Autodesk Inventor part; units mm, degrees
ref_plane "YZ Plane" through (0, 0, 0) normal (1, 0, 0) x (0, 1, 0)
ref_plane "XZ Plane" through (0, 0, 0) normal (0, 1, 0) x (-1, 0, 0)
ref_plane "XY Plane" through (0, 0, 0) normal (0, 0, 1) x (1, 0, 0)
sketch "Sketch1" plane through (0, 0, 0) normal (1, 0, 0) x (0, 1, 0)
  line L0 (13.5, 0) -> (169.5, 0)
  line L1 (183, -13.5) -> (183, -169.5)
  line L2 (169.5, -183) -> (13.5, -183)
  line L3 (0, -169.5) -> (0, -13.5)
  arc A0 (183, -13.5) -> (169.5, 0) centre (169.5, -13.5) ccw
  arc A1 (169.5, -183) -> (183, -169.5) centre (169.5, -169.5) ccw
  arc A2 (0, -169.5) -> (13.5, -183) centre (13.5, -169.5) ccw
  arc A3 (13.5, 0) -> (0, -13.5) centre (13.5, -13.5) ccw
  line L4 (169.5, -13.5) -> (13.5, -13.5)
  line L5 (13.5, -13.5) -> (13.5, -145.5)
  line L6 (37.5, -169.5) -> (169.5, -169.5)
  line L7 (169.5, -169.5) -> (169.5, -13.5)
  line L8 (169.5, -13.5) -> (179.0459, -3.9541) construction
  line L9 (169.5, -169.5) -> (179.0459, -179.0459) construction
  line L10 (13.5, -13.5) -> (3.9541, -3.9541) construction
  line L11 (33.0959, -149.5) -> (0, -149.5) construction
  line L12 (33.5, -149.9041) -> (33.5, -183) construction
  circle A4 centre (6.0754, -6.0754) radius 3 construction
  circle A5 centre (6.0754, -6.0754) radius 1.1
  circle A6 centre (176.9246, -6.0754) radius 3 construction
  circle A7 centre (176.9246, -6.0754) radius 1.1
  circle A8 centre (176.9246, -176.9246) radius 3 construction
  circle A9 centre (176.9246, -176.9246) radius 1.1
  circle A10 centre (33.5, -180) radius 3 construction
  circle A11 centre (33.5, -180) radius 1.1
  circle A12 centre (3, -149.5) radius 3 construction
  circle A13 centre (3, -149.5) radius 1.1
  line L13 (13.5, -169.5) -> (24.5, -158.5) construction
  circle A14 centre (24.5, -158.5) radius 8.1
  line L14 (13.5, -145.5) -> (33.5, -145.5)
  line L15 (37.5, -149.5) -> (37.5, -169.5)
  arc A15 (37.5, -149.5) -> (33.5, -145.5) centre (33.5, -149.5) ccw
  point P0 (0, 0)
  point P1 (37.5, -145.5)
  dimension "d6" = 6
  dimension "d0" = 13.5
  dimension "d1" = 183
  dimension "d2" = 183
  dimension "d3" = 20
  dimension "d4" = 20
  dimension "d5" = 2.2
  dimension "d10" = 16.2
  dimension "d11" = 24.5
  dimension "d12" = 45
  dimension "d13" = 24
  dimension "d14" = 4
extrude "Extrusion1" add sketch "Sketch1" along normal blind 2.5
properties part number "FrontPanelSquishything"
Verification items for the finished model (mm, model axes). A direction names the side the tool comes from. Round coordinates to 2 decimals unless told otherwise and drop trailing zeros. Order: outer loops, then holes, each group sorted by start corner. A loop starts at its lowest first (then second) coordinate and runs counter-clockwise, first axis right, second up.
1) Draft check along Y on faces 1 (the flat face through (0, 90, -172)), 2 (the cylindrical face through (1.2, 28.9, -165.3)), 3 (the cylindrical face through (1.23, 4.06, -179.15)). Enter one of: +Y half, -Y half, draft (parallel to the pull), parting line (faces both ways), or undercut.
Geometry says:
face 1: draft
face 2: undercut
face 3: -Y half
2) Depth check by flat-ended pin: pin 1 (13 mm diameter, centred on y = 24.5, z = -158.5, fed in from +X). Enter the tip coordinate at first touch or a pass-through.
Geometry says:
pin 1: passes through
3) Material ranges on line 1 (Y direction, x = 0.3, z = -16.5); line 2 (Z direction, x = 2.3, y = 126); line 3 (Z direction, x = 1.25, y = 33.5), recorded low to high.
Geometry says:
line 1: y = 0 to 13.5, 169.5 to 183
line 2: z = -183 to -169.5, -13.5 to 0
line 3: z = -183 to -181.1, -178.9 to -145.5, -13.5 to 0
4) Cross-section at D-D, the plane y = 30. Record the cut outline in (x, z).
Geometry says:
outline: (0, -183) - (2.5, -183) - (2.5, -164.45) - (0, -164.45) - close; (0, -152.55) - (2.5, -152.55) - (2.5, -145.5) - (0, -145.5) - close; (0, -13.5) - (2.5, -13.5) - (2.5, 0) - (0, 0) - close
5) Cross-section at A-A, the plane z = -44.5. Record the cut outline in (x, y).
Geometry says:
outline: (0, 0) - (2.5, 0) - (2.5, 13.5) - (0, 13.5) - close; (0, 169.5) - (2.5, 169.5) - (2.5, 183) - (0, 183) - close
6) Cross-section at B-B, the plane y = 134. Record the cut outline in (x, z), plus the area to 3 significant figures.
Geometry says:
outline: (0, -183) - (2.5, -183) - (2.5, -169.5) - (0, -169.5) - close; (0, -13.5) - (2.5, -13.5) - (2.5, 0) - (0, 0) - close
area: 67.5 mm2
7) Tool access check on faces 4 (the cylindrical face through (1.232, 36.297, -146.641)), 5 (the flat face through (2.5, 90, -172)). Record the directions out of +Z, -Z, +X, -X, +Y, -Y that give a thin tool (end or side, any length) a straight path to the whole face; none if there is none.
Geometry says:
face 4: +X, -X
face 5: +Z, -Z, +X, +Y, -Y
8) Cross-section at C-C, the plane x = 1.25. Record the cut outline in (y, z).
Geometry says:
outline: (0, -169.5) arc R13.5 ccw to (13.5, -183) - (169.5, -183) arc R13.5 ccw to (183, -169.5) - (183, -13.5) arc R13.5 ccw to (169.5, 0) - (13.5, 0) arc R13.5 ccw to (0, -13.5) - close; hole circle Ø2.2 at (3, -149.5); hole circle Ø2.2 at (6.08, -6.08); hole (13.5, -145.5) - (33.5, -145.5) arc R4 cw to (37.5, -149.5) - (37.5, -169.5) - (169.5, -169.5) - (169.5, -13.5) - (13.5, -13.5) - close; hole circle Ø16.2 at (24.5, -158.5); hole circle Ø2.2 at (33.5, -180); hole circle Ø2.2 at (176.92, -176.92); hole circle Ø2.2 at (176.92, -6.08)
